from build123d import *

# Parameters (mm, degrees)
BOSS_EXTRUDE1_DEPTH       = 5.842
BOSS_EXTRUDE2_DEPTH       = 5.842
SKETCH19_R                = 2.159
CUT_EXTRUDE1_DEPTH        = 2.54
F_6_32_TAPPED_HOLE1_D     = 2.7051
F_6_32_TAPPED_HOLE1_DEPTH = 0.635


with BuildPart() as part:
    # Sketch1 → Boss-Extrude1 (new body)
    with BuildSketch(Plane.XY):
        Polygon((-3.034436618, 16.25018662), (-3.034436618, -2.29181338), (6.617563382, -2.29181338), (6.617563382, 16.25018662), (5.982563382, 16.25018662), (5.982563382, -1.52981338), (-2.399436618, -1.52981338), (-2.399436618, 16.25018662), align=None)
    extrude(amount=BOSS_EXTRUDE1_DEPTH)

    # Sketch15 → Boss-Extrude2 (add, through all)
    with BuildSketch(Plane.XY):
        with BuildLine():
            Line((6.617563382, -2.29181338), (-3.034436618, -2.29181338))
            ThreePointArc((-3.034436618, -2.29181338), (1.791563382, -2.477704159), (6.617563382, -2.29181338))
        make_face()
    extrude(amount=BOSS_EXTRUDE2_DEPTH)

    # Sketch19 → Cut-Extrude1 (cut)
    with BuildSketch(Plane(origin=(6.617563382, 0, 0), x_dir=(0, 0, -1), z_dir=(1, 0, 0))):
        with Locations((-2.921, 11.17018662)):
            Circle(SKETCH19_R)
    extrude(amount=-CUT_EXTRUDE1_DEPTH, mode=Mode.SUBTRACT)

    # #6-32 Tapped Hole1
    with Locations(Plane.ZY.offset(3.034436618)):
        with Locations((2.921, 11.17018662)):
            Hole(F_6_32_TAPPED_HOLE1_D / 2, depth=F_6_32_TAPPED_HOLE1_DEPTH)


solid = part.part
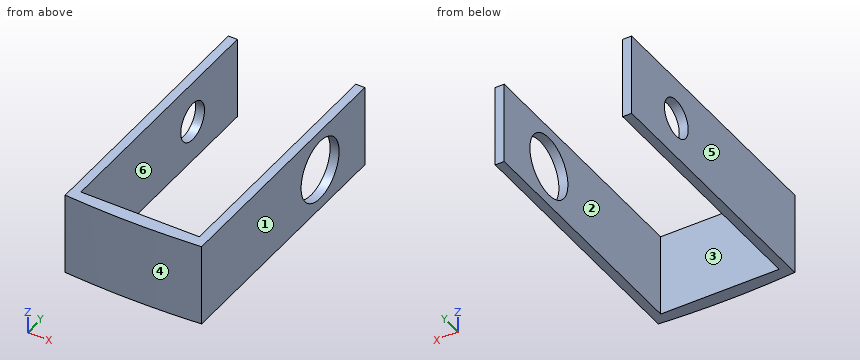
Could you check a few things on this model? Use its own coordinates, in mm. Face numbers are marked on the shaded views. A direction names the side the tool comes from. Coordinates: 2 decimals unless noted, no trailing zeros. Order: outer loops, then holes, each group sorted by start corner. A loop starts at its lowest first (then second) coordinate and runs counter-clockwise, first axis right, second up.
Q1. Suppose I cut it at A-A on y = 13.75. Please give me the cut outline in (x, z), and give its area (3 significant figures).
Q2. Suppose I cut it at C-C on z = 1.3. Please give me the cut outline in (x, y), and give its area (3 significant figures).
Q3. Suppose I cut it at B-B on z = 2.5. Please give me the cut outline in (x, y), and give its area (3 significant figures).
Q4. Thinking about a two-plate mould opening in X: for the marked faces 1, 2, 3 and 4, which applies, released by +X, released by -X, zero draft, split by the parting line, or undercut?
Q5. Which directions (+Z, -Z, +X, -X, +Y, -Y) give clear straight access to the entire face, cutting with the end or side of a thin tool? Please do the marked faces 5 and 6.
Q6. Suppose I cut it at D-D on y = 11.5. Please give me the cut outline in (x, z).
Q7. Please list where these lines run through material, in increasing order: L1, parallel to X at y = 6.75, z = 4.3; L2, parallel to Y at x = 2.5, z = 5.5; L3, parallel to Y at x = -1.5, z = 0.35.
Answer:
1. outline: (-3.03, 0) - (-2.4, 0) - (-2.4, 5.84) - (-3.03, 5.84) - close; (5.98, 0) - (6.62, 0) - (6.62, 5.84) - (5.98, 5.84) - close
1. area: 7.42 mm2
2. outline: (-3.03, -2.29) arc R62.74 ccw to (6.62, -2.29) - (6.62, 9.74) - (5.98, 9.74) - (5.98, -1.53) - (-2.4, -1.53) - (-2.4, 16.25) - (-3.03, 16.25) - close; (5.98, 12.6) - (6.62, 12.6) - (6.62, 16.25) - (5.98, 16.25) - close
2. area: 29.3 mm2
3. outline: (-3.03, -2.29) arc R62.74 ccw to (6.62, -2.29) - (6.62, 9.05) - (5.98, 9.05) - (5.98, -1.53) - (-2.4, -1.53) - (-2.4, 9.88) - (-3.03, 9.88) - close; (-3.03, 12.46) - (-2.4, 12.46) - (-2.4, 16.25) - (-3.03, 16.25) - close; (5.98, 13.29) - (6.62, 13.29) - (6.62, 16.25) - (5.98, 16.25) - close
3. area: 26.8 mm2
4. face 1: released by +X
4. face 2: undercut
4. face 3: undercut
4. face 4: split by the parting line
5. face 5: +Z, -Z, -X, +Y, -Y
5. face 6: +Z, -Z, +Y
6. outline: (-3.03, 0) - (-2.4, 0) - (-2.4, 1.61) - (-3.03, 1.61) - close; (-3.03, 4.23) - (-2.4, 4.23) - (-2.4, 5.84) - (-3.03, 5.84) - close; (5.98, 0) - (6.62, 0) - (6.62, 0.79) - (5.98, 0.79) - close; (5.98, 5.05) - (6.62, 5.05) - (6.62, 5.84) - (5.98, 5.84) - close
7. L1: x = -3.03 to -2.4, 5.98 to 6.62
7. L2: y = -2.47 to -1.53
7. L3: y = -2.39 to -1.53
